from build123d import *

# Parameters (mm, degrees)
F0_W     = 304.8
F0_H     = 88.9
F1_DEPTH = 17.78
F2_W     = 152.4
F2_H     = 76.2
F3_DEPTH = 25.4
F4_R     = 38.1
F5_DEPTH = 25.4
F6_W     = 10.16
F6_H     = 10.16
F7_DEPTH = 128.9815305102


with BuildPart() as f1:
    # F0 (on Top) → F1 (new body)
    with BuildSketch(Plane.XY):
        with Locations((-65.4162000656, -0.3342888534)):
            Rectangle(F0_W, F0_H)
    extrude(amount=F1_DEPTH)

    # F2 (on face) → F3 (cut)
    with BuildSketch(Plane.XY.offset(17.78)):
        with Locations((10.7837999344, 6.0157111466)):
            Rectangle(F2_W, F2_H)
    extrude(amount=-F3_DEPTH, mode=Mode.SUBTRACT)

    # F4 (on face) → F5 (cut)
    with BuildSketch(Plane.XY.offset(17.78)):
        with Locations((-152.0220041275, 0)):
            Circle(F4_R)
    extrude(amount=-F5_DEPTH, mode=Mode.SUBTRACT)

    # F6 (on Right) → F7 (cut, up to face)
    with BuildSketch(Plane.YZ):
        with Locations((-24.4778353107, 5.08)):
            Rectangle(F6_W, F6_H)
    extrude(amount=-F7_DEPTH, mode=Mode.SUBTRACT)


solid = f1.part
Geometry check sheet. Reference: the model listing, model coordinates, mm. A direction names the side the tool comes from. Give positions to 0.01 mm unless a question says otherwise; leave off trailing zeros. Order: outer loops, then holes, each group sorted by start corner. A loop starts at its lowest first (then second) coordinate and runs counter-clockwise, first axis right, second up. Notation, with made-up numbers: (89, 81) - (102, 81) arc R32 ccw to (102, 107) - close; hole circle Ø6 at (23, 69). An arc over 180 degrees is marked (long way). Answer as a JSON object with one key per item and string values.
(1) Cross-section at C-C (x = -150). Record the cut outline in (y, z), then the cut area to 3 significant figures.
Report:
{"outline": "(-44.78, 0) - (-38.05, 0) - (-38.05, 17.78) - (-44.78, 17.78) - close; (38.05, 0) - (44.12, 0) - (44.12, 17.78) - (38.05, 17.78) - close", "area": "228 mm^2"}
(2) Draft check along Y on faces 1 (the flat face through (-65.416, 5, 9)), 2 (the flat face through (-96, -25, 10.16)), 3 (the flat face through (10, -32.084, 9)). Enter one of: released by +Y, released by -Y, zero draft, split by the parting line, or undercut.
Report:
{"face 1": "zero draft", "face 2": "undercut", "face 3": "released by +Y"}
(3) Tool access check on faces 4 (the cylindrical face through (-160.281, -37.194, 9.014)), 5 (the flat face through (-92, -19.398, 5)). Record the directions out of +Z, -Z, +X, -X, +Y, -Y that give a thin tool (end or side, any length) a straight path to the whole face; none if there is none.
Report:
{"face 4": "+Z, -Z", "face 5": "-Z, +X"}
(4) Material ranges on line 1 (X direction, y = 0, z = 7); line 2 (Y direction, x = -43, z = 14.75); line 3 (X direction, y = 25, z = 8), recorded low to high.
Report:
{"line 1": "-217.82 to -190.12, -113.92 to -65.42", "line 2": "-44.78 to -32.08", "line 3": "-217.82 to -180.77, -123.27 to -65.42"}
(5) Cross-section at D-D (x = -92). Record the cut outline in (y, z).
Report:
{"outline": "(-44.78, 0) - (-29.56, 0) - (-29.56, 10.16) - (-19.4, 10.16) - (-19.4, 0) - (44.12, 0) - (44.12, 17.78) - (-44.78, 17.78) - close"}
(6) Depth check by flat-ended pin: pin 1 Ø9 at (y, z) = (22.5, 9.5) entering from +X; pin 2 Ø11 at (x, y) = (-82, -25) entering from -Z. Enter the tip coordinate at first touch or a pass-through.
Report:
{"pin 1": "x = -65.42", "pin 2": "z = 0"}
(7) Cross-section at B-B (z = 12.75). Record the cut outline in (x, y).
Report:
{"outline": "(-217.82, -44.78) - (86.98, -44.78) - (86.98, -32.08) - (-65.42, -32.08) - (-65.42, 44.12) - (-217.82, 44.12) - close; hole circle Ø76.2 at (-152.02, 0)"}
(8) Cross-section at A-A (y = 0). Record the cut outline in (x, z), then the cut area to 3 significant figures.
Report:
{"outline": "(-217.82, 0) - (-190.12, 0) - (-190.12, 17.78) - (-217.82, 17.78) - close; (-113.92, 0) - (-65.42, 0) - (-65.42, 17.78) - (-113.92, 17.78) - close", "area": "1,350 mm^2"}
